Part model, mm, in its own coordinate system. Face numbers are marked on the shaded views. A direction names the side the tool comes from. Coordinates: 2 decimals unless noted, no trailing zeros. Write each loop counter-clockwise with the first axis right and the second up, starting at its lowest first coordinate (ties: lowest second). Pieces come first, ordered by that corner, then holes. Notation, with made-up numbers: (63.5, 27.25) - (67.5, 27.25) arc R29 cw to (67.5, 53.25) - close; hole circle Ø10 at (-8, -39). An arc over 180 degrees is marked (long way). Write each question's results on one line, items separated by ' | '.
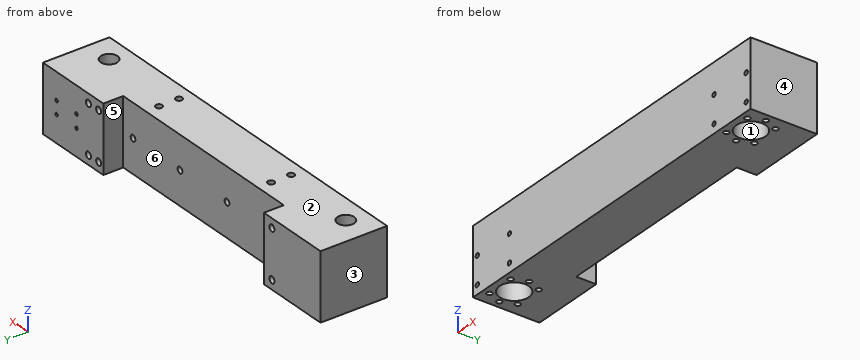
from build123d import *

# Parameters (mm, degrees)
SKETCH1_R              = 14
SKETCH1_R_2            = 2.6035
BOSS_EXTRUDE1_DEPTH    = 63.5
SKETCH2_R              = 3.175
CUT_EXTRUDE1_DEPTH     = 19.05
CUT_EXTRUDE3_START     = -63.5
CUT_EXTRUDE3_DEPTH     = 6.35
BOSS_EXTRUDE2_START    = -32
SKETCH3_R              = 14
SKETCH3_R_2            = 8
BOSS_EXTRUDE2_DEPTH    = 31.5
SKETCH4_R              = 1.5875
CUT_EXTRUDE4_DEPTH     = 6.35
BOSS_EXTRUDE3_START    = -50.8
SKETCH5_R              = 2.6035
BOSS_EXTRUDE3_DEPTH    = 50.8
CUT_EXTRUDE5_DEPTH     = 6.35
CUT_EXTRUDE6_START     = -6.35
CUT_EXTRUDE6_OUTLINE_R = 3.175
CUT_EXTRUDE6_DEPTH     = 6.35


# Read off the part's stored shape, not the designer's step: Cut-Extrude6
with BuildPart() as part:
    # Sketch1 → Boss-Extrude1 (new body)
    with BuildSketch(Plane.XY):
        Polygon((100.125, 63.5), (100.125, 44.5), (-104.875, 44.5), (-104.875, 63.5), (-177.125, 63.5), (-177.125, 0), (177.125, 0), (177.125, 63.5), align=None)
        with Locations((-151.3, 20)):
            Circle(SKETCH1_R, mode=Mode.SUBTRACT)
        with Locations((150.95, 20)):
            Circle(SKETCH1_R, mode=Mode.SUBTRACT)
        with Locations((-164.735028843, 6.564971157)):
            Circle(SKETCH1_R_2, mode=Mode.SUBTRACT)
        with Locations((-137.864971157, 6.564971157)):
            Circle(SKETCH1_R_2, mode=Mode.SUBTRACT)
        with Locations((-132.3, 20)):
            Circle(SKETCH1_R_2, mode=Mode.SUBTRACT)
        with Locations((-137.864971157, 33.435028843)):
            Circle(SKETCH1_R_2, mode=Mode.SUBTRACT)
        with Locations((-170.3, 20)):
            Circle(SKETCH1_R_2, mode=Mode.SUBTRACT)
        with Locations((-164.735028843, 33.435028843)):
            Circle(SKETCH1_R_2, mode=Mode.SUBTRACT)
        with Locations((137.514971157, 6.564971157)):
            Circle(SKETCH1_R_2, mode=Mode.SUBTRACT)
        with Locations((164.385028843, 6.564971157)):
            Circle(SKETCH1_R_2, mode=Mode.SUBTRACT)
        with Locations((169.95, 20)):
            Circle(SKETCH1_R_2, mode=Mode.SUBTRACT)
        with Locations((164.385028843, 33.435028843)):
            Circle(SKETCH1_R_2, mode=Mode.SUBTRACT)
        with Locations((131.95, 20)):
            Circle(SKETCH1_R_2, mode=Mode.SUBTRACT)
        with Locations((137.514971157, 33.435028843)):
            Circle(SKETCH1_R_2, mode=Mode.SUBTRACT)
    extrude(amount=BOSS_EXTRUDE1_DEPTH)

    # Sketch2 → Cut-Extrude1 (cut)
    with BuildSketch(Plane(origin=(0, 63.5, 0), x_dir=(1, 0, 0), z_dir=(0, 1, 0))):
        with Locations(Location((119.125, -54.75, 0), (0, 0, 180))):
            Circle(SKETCH2_R)
        with Locations(Location((106.125, -54.75, 0), (0, 0, 180))):
            Circle(SKETCH2_R)
        with Locations(Location((119.125, -8.75, 0), (0, 0, 180))):
            Circle(SKETCH2_R)
        with Locations(Location((106.125, -8.75, 0), (0, 0, 180))):
            Circle(SKETCH2_R)
        with Locations(Location((-115.125, -54.75, 0), (0, 0, 180))):
            Circle(SKETCH2_R)
        with Locations(Location((-115.125, -8.75, 0), (0, 0, 180))):
            Circle(SKETCH2_R)
    extrude(amount=-CUT_EXTRUDE1_DEPTH, mode=Mode.SUBTRACT)

    # Sketch2<3> → Cut-Extrude3 (cut)
    with BuildSketch(Plane(origin=(0, 63.5, 0), x_dir=(1, 0, 0), z_dir=(0, 1, 0)).offset(CUT_EXTRUDE3_START)):
        with BuildLine():
            ThreePointArc((169.525, -34.65), (171.625, -36.75), (173.725, -34.65))
            ThreePointArc((173.725, -34.65), (171.625, -32.55), (169.525, -34.65))
        make_face()
        with BuildLine():
            ThreePointArc((128.525, -34.65), (130.625, -36.75), (132.725, -34.65))
            ThreePointArc((132.725, -34.65), (130.625, -32.55), (128.525, -34.65))
        make_face()
        with BuildLine():
            ThreePointArc((128.525, -8.65), (130.625, -10.75), (132.725, -8.65))
            ThreePointArc((132.725, -8.65), (130.625, -6.55), (128.525, -8.65))
        make_face()
        with BuildLine():
            ThreePointArc((169.525, -8.65), (171.625, -10.75), (173.725, -8.65))
            ThreePointArc((173.725, -8.65), (171.625, -6.55), (169.525, -8.65))
        make_face()
        with BuildLine():
            ThreePointArc((-132.725, -34.65), (-130.625, -36.75), (-128.525, -34.65))
            ThreePointArc((-128.525, -34.65), (-130.625, -32.55), (-132.725, -34.65))
        make_face()
        with BuildLine():
            ThreePointArc((-132.725, -8.65), (-130.625, -10.75), (-128.525, -8.65))
            ThreePointArc((-128.525, -8.65), (-130.625, -6.55), (-132.725, -8.65))
        make_face()
        with BuildLine():
            ThreePointArc((-173.725, -8.65), (-171.625, -10.75), (-169.525, -8.65))
            ThreePointArc((-169.525, -8.65), (-171.625, -6.55), (-173.725, -8.65))
        make_face()
        with BuildLine():
            ThreePointArc((-173.725, -34.65), (-171.625, -36.75), (-169.525, -34.65))
            ThreePointArc((-169.525, -34.65), (-171.625, -32.55), (-173.725, -34.65))
        make_face()
    extrude(amount=CUT_EXTRUDE3_DEPTH, mode=Mode.SUBTRACT)

    # Sketch3 → Boss-Extrude2 (add)
    # profile 1 of 2: a face of its own
    with BuildSketch(Plane(origin=(0, 0, 0), x_dir=(-1, 0, 0), z_dir=(0, 0, -1)).offset(BOSS_EXTRUDE2_START)):
        with Locations(Location((-150.95, 20, 0), (0, 0, 180))):
            Circle(SKETCH3_R)
        with Locations(Location((-150.95, 20, 0), (0, 0, 180))):
            Circle(SKETCH3_R_2, mode=Mode.SUBTRACT)
    # profile 2 of 2: a face of its own
    with BuildSketch(Plane(origin=(0, 0, 0), x_dir=(-1, 0, 0), z_dir=(0, 0, -1)).offset(BOSS_EXTRUDE2_START)):
        with Locations(Location((151.3, 20, 0), (0, 0, 180))):
            Circle(SKETCH3_R)
        with Locations(Location((151.3, 20, 0), (0, 0, 180))):
            Circle(SKETCH3_R_2, mode=Mode.SUBTRACT)
    extrude(amount=-BOSS_EXTRUDE2_DEPTH)

    # Sketch4 → Cut-Extrude4 (cut)
    with BuildSketch(Plane(origin=(0, 63.5, 0), x_dir=(1, 0, 0), z_dir=(0, 1, 0))):
        with Locations(Location((159.775, -38.075, 0), (0, 0, 180))):
            Circle(SKETCH4_R)
        with Locations(Location((159.775, -25.425, 0), (0, 0, 180))):
            Circle(SKETCH4_R)
        with Locations(Location((134.375, -25.425, 0), (0, 0, 180))):
            Circle(SKETCH4_R)
        with Locations(Location((134.375, -38.075, 0), (0, 0, 180))):
            Circle(SKETCH4_R)
    extrude(amount=-CUT_EXTRUDE4_DEPTH, mode=Mode.SUBTRACT)

    # Sketch5 → Boss-Extrude3 (add)
    with BuildSketch(Plane.XY.offset(63.5).offset(BOSS_EXTRUDE3_START)):
        with Locations((131.95, 20)):
            Circle(SKETCH5_R)
        with Locations((137.514971157, 6.564971157)):
            Circle(SKETCH5_R)
        with Locations((164.385028843, 6.564971157)):
            Circle(SKETCH5_R)
        with Locations((169.95, 20)):
            Circle(SKETCH5_R)
        with Locations((164.385028843, 33.435028843)):
            Circle(SKETCH5_R)
        with Locations((137.514971157, 33.435028843)):
            Circle(SKETCH5_R)
        with Locations((-137.864971157, 6.564971157)):
            Circle(SKETCH5_R)
        with Locations((-132.3, 20)):
            Circle(SKETCH5_R)
        with Locations((-137.864971157, 33.435028843)):
            Circle(SKETCH5_R)
        with Locations((-164.735028843, 6.564971157)):
            Circle(SKETCH5_R)
        with Locations((-170.3, 20)):
            Circle(SKETCH5_R)
        with Locations((-164.735028843, 33.435028843)):
            Circle(SKETCH5_R)
    extrude(amount=BOSS_EXTRUDE3_DEPTH)

    # Sketch6 → Cut-Extrude5 (cut)
    with BuildSketch(Plane(origin=(0, 44.5, 0), x_dir=(1, 0, 0), z_dir=(0, 1, 0))):
        with BuildLine():
            ThreePointArc((87.625, -34.925), (90.625, -31.925), (87.625, -28.925))
            ThreePointArc((87.625, -28.925), (84.625, -31.925), (87.625, -34.925))
        make_face()
        with BuildLine():
            ThreePointArc((27.625, -34.925), (30.625, -31.925), (27.625, -28.925))
            ThreePointArc((27.625, -28.925), (24.625, -31.925), (27.625, -34.925))
        make_face()
        with BuildLine():
            ThreePointArc((-32.3698, -34.925), (-29.3698, -31.925), (-32.3698, -28.925))
            ThreePointArc((-32.3698, -28.925), (-35.3698, -31.925), (-32.3698, -34.925))
        make_face()
        with BuildLine():
            ThreePointArc((-92.3646, -34.925), (-89.3646, -31.925), (-92.3646, -28.925))
            ThreePointArc((-92.3646, -28.925), (-95.3646, -31.925), (-92.3646, -34.925))
        make_face()
    extrude(amount=-CUT_EXTRUDE5_DEPTH, mode=Mode.SUBTRACT)

    # Cut-Extrude6 outline → Cut-Extrude6 (cut)
    with BuildSketch(Plane.XY.offset(63.5).offset(CUT_EXTRUDE6_START)):
        with Locations((-71.6887, 31.8)):
            Circle(CUT_EXTRUDE6_OUTLINE_R)
        with Locations((71.3387, 12.75)):
            Circle(CUT_EXTRUDE6_OUTLINE_R)
        with Locations((71.3387, 31.8)):
            Circle(CUT_EXTRUDE6_OUTLINE_R)
        with Locations((-71.6887, 12.75)):
            Circle(CUT_EXTRUDE6_OUTLINE_R)
    extrude(amount=CUT_EXTRUDE6_DEPTH, mode=Mode.SUBTRACT)


solid = part.part
(1) Saw through at B-B on x = 150.95. Write the cut outline in (y, z).
Return value:
outline: (0, 0) - (6, 0) - (6, 32) - (12, 32) - (12, 63.5) - (0, 63.5) - close; (28, 32) - (34, 32) - (34, 0) - (63.5, 0) - (63.5, 63.5) - (28, 63.5) - close
(2) Wall check: line 1 (X direction, y = 20.5, z = 46.5) (3 decimals); line 2 (X direction, y = 13, z = 56.5) (3 decimals); line 3 (X direction, y = 54.5, z = 13) (3 decimals). Give the ranges that are in metal, low to high. Write a range as from..to.
Return value:
line 1: x = -177.125..-159.284, -143.316..142.966, 158.934..177.125 | line 2: x = -177.125..-155.173, -147.427..147.077, 154.823..177.125 | line 3: x = -177.125..-104.875, 100.125..177.125
(3) Saw through at A-A on y = 50.5. Write the cut outline in (x, z) (3 decimals).
Return value:
outline: (-177.125, 0) - (-104.875, 0) - (-104.875, 63.5) - (-177.125, 63.5) - close; (100.125, 0) - (177.125, 0) - (177.125, 63.5) - (100.125, 63.5) - close; hole circle Ø6.35 at (-115.125, 8.75); hole circle Ø6.35 at (-115.125, 54.75); hole circle Ø6.35 at (106.125, 8.75); hole circle Ø6.35 at (106.125, 54.75); hole circle Ø6.35 at (119.125, 8.75); hole circle Ø6.35 at (119.125, 54.75)
(4) Flat gauge pins, fed straight in: P1, Ø1.9, axis at x = -71, y = 30.5, coming from the +Z side; P2, Ø1.3, axis at x = -131.5, z = 9.5, coming from the -Y side; P3, Ø2.5, axis at x = -138.5, y = 6, coming from the -Z side. Where does each tip first touch, or does it go through?
Return value:
P1: stops at z = 57.15 | P2: stops at y = 6.35 | P3: stops at z = 12.7
(5) 3-axis set-ups, long thin cutter, end or side, ignore diameter. For the marked faces 1 and 2: which of +Z, -Z, +X, -X, +Y, -Y reach the whole face in a straight line?
Return value:
face 1: -Z | face 2: +Z, +X, -X, +Y, -Y
(6) Two-plate mould, pull along X, no slides. Class the marked faces 3, 4, 5 and 6: released by +X, released by -X, zero draft, split by the parting line, or undercut.
Return value:
face 3: released by -X | face 4: released by +X | face 5: undercut | face 6: undercut
